The listing builds one solid part. Answer for the finished solid, in the listing's coordinates (mm). A direction names the side the tool comes from. Coordinates: 2 decimals unless noted, no trailing zeros. Loops run counter-clockwise (first coordinate to the right, second up) from the corner with the lowest first, then second, coordinate; pieces in that order, holes last. Notation, with made-up numbers: (-8, -22.75) - (4, -22.75) arc R19 ccw to (4, 9.25) - close; hole circle Ø11 at (67.25, -35.75). An arc over 180 degrees is marked (long way). One line per question, with ' | ' between items.
from build123d import *

# Parameters (mm, degrees)
SKETCH_1_R      = 19
EXTRUDE_1_DEPTH = 4
SKETCH_2_R      = 8
EXTRUDE_2_DEPTH = 8
SKETCH_3_R      = 14
EXTRUDE_3_DEPTH = 14
SKETCH_4_R      = 11
EXTRUDE_4_DEPTH = 2
SKETCH_5_R      = 14
EXTRUDE_5_DEPTH = 7
SKETCH_6_W      = 30
SKETCH_6_H      = 34
EXTRUDE_6_DEPTH = 40


with BuildPart() as part:
    # 草图1 → 凸台-拉伸1 (new body)
    with BuildSketch(Plane.XY):
        Circle(SKETCH_1_R)
    extrude(amount=EXTRUDE_1_DEPTH)

    # 草图2 → 凸台-拉伸2 (add)
    with BuildSketch(Plane.XY.offset(4)):
        Circle(SKETCH_2_R)
    extrude(amount=EXTRUDE_2_DEPTH)

    # 草图3 → 凸台-拉伸3 (add)
    with BuildSketch(Plane.XY.offset(12)):
        Circle(SKETCH_3_R)
    extrude(amount=EXTRUDE_3_DEPTH)

    # 草图4 → 凸台-拉伸4 (add)
    with BuildSketch(Plane.XY.offset(26)):
        Circle(SKETCH_4_R)
    extrude(amount=EXTRUDE_4_DEPTH)

    # 草图5 → 凸台-拉伸5 (add)
    with BuildSketch(Plane.XY.offset(28)):
        Circle(SKETCH_5_R)
    extrude(amount=EXTRUDE_5_DEPTH)

    # 草图6 → 凸台-拉伸6 (add)
    with BuildSketch(Plane.XY.offset(35)):
        Rectangle(SKETCH_6_W, SKETCH_6_H)
    extrude(amount=EXTRUDE_6_DEPTH)


solid = part.part
Item 1: Find the intervals of material crossed by line 1 (Z direction, x = 13, y = 1.5); line 2 (Z direction, x = 14.5, y = 2.5); line 3 (Z direction, x = 8, y = 1.5), in increasing order. Write a range as [from, to].
Taken from the geometry:
line 1: z = [0, 4], [12, 26], [28, 75] | line 2: z = [0, 4], [35, 75] | line 3: z = [0, 4], [12, 75]
Item 2: Find section D-D, the plane z = 11. Write down the section's boundary in (x, y), plus the area to 3 significant figures.
Taken from the geometry:
outline: circle Ø16 at (0, 0) | area: 201 mm2
Item 3: Each of these flat-tipped pins is pushed along its axis until it touches: pin 1 Ø1 at (y, z) = (-2.5, 64.5) entering from +X; pin 2 Ø2 at (y, z) = (6, 23) entering from +X; pin 3 Ø9 at (x, z) = (7, 54) entering from -Y. Where does it stop, or does it pass through?
Taken from the geometry:
pin 1: stops at x = 15 | pin 2: stops at x = 13.08 | pin 3: stops at y = -17
Item 4: The mould has two halves that part along Z. Classify faces 1 (the face through (0, 0, 75)), 2 (the face through (6, -6, 12)), 3 (the face through (12.932, -5.362, 18.902)), 4 (the face through (0, 17, 55)): pulls with the +Z half, pulls with the -Z half, needs draft (parallel to the pull), parting line crosses it, or undercut.
Taken from the geometry:
face 1: pulls with the +Z half | face 2: undercut | face 3: undercut | face 4: needs draft
Item 5: Find section A-A, the plane y = 15.5. Write down the section's boundary in (x, z).
Taken from the geometry:
outline: (-15, 35) - (15, 35) - (15, 75) - (-15, 75) - close; (-10.99, 0) - (10.99, 0) - (10.99, 4) - (-10.99, 4) - close
Item 6: Find section B-B, the plane x = 0. Write down the section's boundary in (y, z).
Taken from the geometry:
outline: (-19, 0) - (19, 0) - (19, 4) - (8, 4) - (8, 12) - (14, 12) - (14, 26) - (11, 26) - (11, 28) - (14, 28) - (14, 35) - (17, 35) - (17, 75) - (-17, 75) - (-17, 35) - (-14, 35) - (-14, 28) - (-11, 28) - (-11, 26) - (-14, 26) - (-14, 12) - (-8, 12) - (-8, 4) - (-19, 4) - close
Item 7: Which of the six approach directions +Z, -Z, +X, -X, +Y, -Y give full straight-line access (tool end or side, diameter ignored) to faces 5 (the face through (8.767, -16.856, 1.972)), 6 (the face through (-15, 0, 55)), 7 (the face through (0, -17, 55)), 8 (the face through (8.2, 0.3, 4)), 9 (the face through (15, 0, 55))?
Taken from the geometry:
face 5: -Z | face 6: +Z, -X, +Y, -Y | face 7: +Z, +X, -X, -Y | face 8: none | face 9: +Z, +X, +Y, -Y
Item 8: Find section C-C, the plane y = 0. Write down the section's boundary in (x, z).
Taken from the geometry:
outline: (-19, 0) - (19, 0) - (19, 4) - (8, 4) - (8, 12) - (14, 12) - (14, 26) - (11, 26) - (11, 28) - (14, 28) - (14, 35) - (15, 35) - (15, 75) - (-15, 75) - (-15, 35) - (-14, 35) - (-14, 28) - (-11, 28) - (-11, 26) - (-14, 26) - (-14, 12) - (-8, 12) - (-8, 4) - (-19, 4) - close
